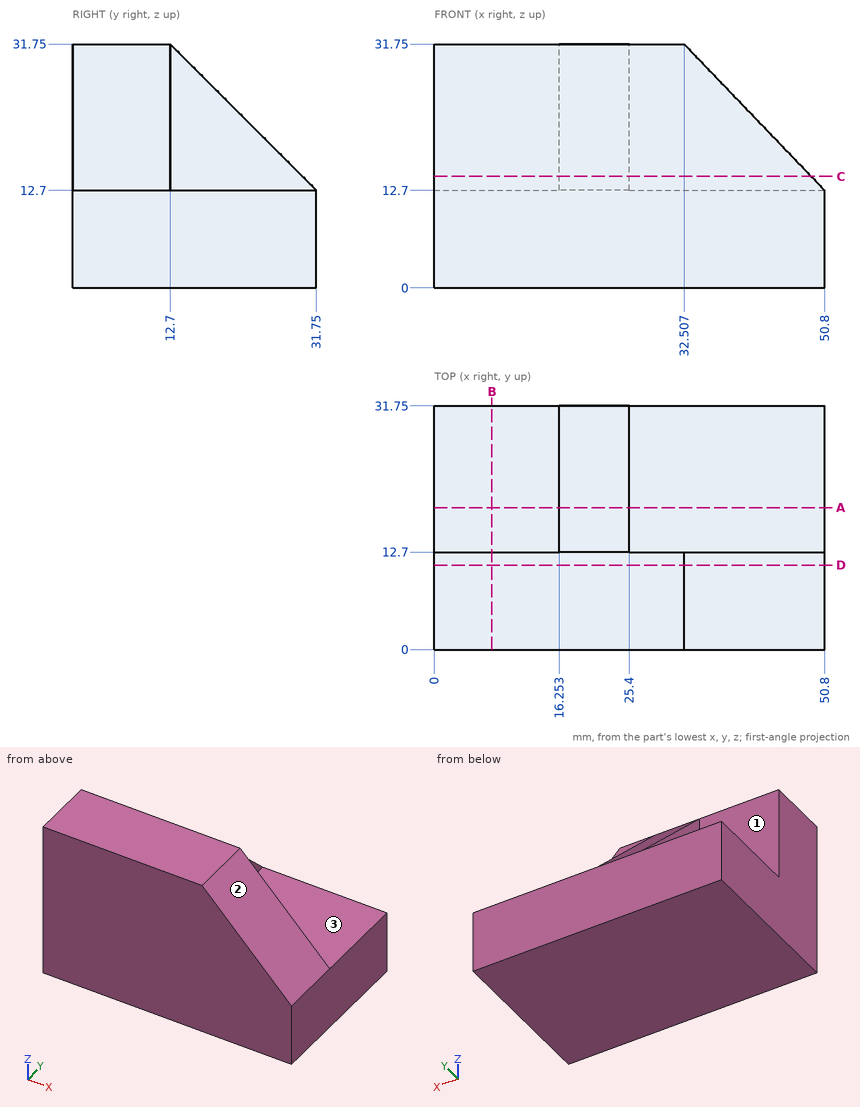
Can you work these out from the drawing? Everything is in mm from the part's minimum corner. A direction names the side the tool comes from. Coordinates: 2 decimals unless noted, no trailing zeros. Write each loop counter-clockwise with the first axis right and the second up, starting at its lowest first coordinate (ties: lowest second). Pieces come first, ordered by that corner, then holes. Notation, with made-up numbers: (89.5, 55) -> (97.5, 55) arc R23 cw to (97.5, 72) -> close; hole circle Ø3 at (-37.5, -32). An arc over 180 degrees is marked (long way). Write item = value, one per line.
(1) Imagine slicing it at D-D (y = 11). Please give me the cut outline in (x, z).
Verdict:
outline = (0, 0) -> (50.8, 0) -> (50.8, 12.7) -> (32.51, 31.75) -> (0, 31.75) -> close
(2) Imagine slicing it at C-C (z = 14.5). Please give me the cut outline in (x, y).
Verdict:
outline = (0, 0) -> (49.07, 0) -> (49.07, 12.7) -> (25.4, 12.7) -> (25.4, 29.95) -> (16.25, 29.95) -> (16.25, 12.7) -> (0, 12.7) -> close
(3) For pin 1 (18 mm diameter, centred on x = 10.5, z = 18, fed in from +Y); pin 2 (5 mm diameter, centred on x = 7.5, z = 17, fed in from +Y); pin 3 (9.5 mm diameter, centred on y = 20.5, z = 26.5, fed in from -X); pin 4 (1.5 mm diameter, centred on x = 43.5, y = 18.5, fed in from +Z), each with a flat end and sliding along its axis, tell me the tip position at first contact or that it passes through.
Verdict:
pin_1 = 31.75
pin_2 = 12.7
pin_3 = 16.25
pin_4 = 12.7
(4) If I drill on probe 1 along Y at (x, z) = (16, 29); probe 2 along X at (y, z) = (14.5, 16), over which ranges is the centre line in solid material (lowest first)?
Verdict:
probe_1 = 0 to 12.7
probe_2 = 16.25 to 25.4
(5) On a 3-axis mill with a long thin cutter (end or side, diameter ignored), from which of +Z, -Z, +X, -X, +Y, -Y can I reach the whole of each face in a straight line? I mean the marked faces 1, 2 and 3. Say none if no direction works.
Verdict:
face_1 = +Z, -X, +Y
face_2 = +Z, +X, +Y, -Y
face_3 = +Z, +X, +Y
(6) Imagine slicing it at A-A (y = 18.5). Please give me the cut outline in (x, z), and give its area (3 significant figures).
Verdict:
outline = (0, 0) -> (50.8, 0) -> (50.8, 12.7) -> (25.4, 12.7) -> (25.4, 25.95) -> (16.25, 25.95) -> (16.25, 12.7) -> (0, 12.7) -> close
area = 766 mm^2
(7) Imagine slicing it at B-B (x = 7.5). Please give me the cut outline in (y, z), and give its area (3 significant figures).
Verdict:
outline = (0, 0) -> (31.75, 0) -> (31.75, 12.7) -> (12.7, 12.7) -> (12.7, 31.75) -> (0, 31.75) -> close
area = 645 mm^2
